Source: CAD feature listing. Evaluate the final solid. Frame: model axes, mm. A direction names the side the tool comes from. Give positions to 0.01 mm unless a question says otherwise; leave off trailing zeros. Order: outer loops, then holes, each group sorted by start corner. A loop starts at its lowest first (then second) coordinate and runs counter-clockwise, first axis right, second up. Notation, with made-up numbers: (38.25, 72.25) - (62.25, 72.25) arc R13 ccw to (62.25, 81.25) - close; hole circle Ø9 at (-36.5, -2.5). An arc over 180 degrees is marked (long way). Write each question's results on one line, items separated by ' | '. Start each with the question number.
Item 1: Set-up query: faces 4 (the cylindrical face through (-41.205, 1.768, 26.863)), 5 (the flat face through (0, -5, -48)), 6 (the cylindrical face through (1.245, -2.465, 53.502)). Return all of +Z, -Z, +X, -X, +Y, -Y with unobstructed straight access to the full face (end or side cutting, diameter ignored); none if empty.
Item 2: Section C-C on z = -50.5. Output: boundary loops of the cut face in (x, y), and give its area (3 significant figures).
Item 3: Mould query, pull axis X, two halves, no side actions, for faces 1 (the cylindrical face through (1.245, -2.465, -47.498)), 2 (the flat face through (0, -5, 53)), 3 (the cylindrical face through (-40.56, -2.46, 24.55)). Classes: released by +X, released by -X, zero draft, split by the parting line, or undercut.
Item 4: Section D-D on x = -31.5. Output: boundary loops of the cut face in (y, z).
Item 5: Contact query for flat-ended pins moving along their axis: pin 1 Ø4.5 at (x, z) = (43.73, -25.25) entering from -Y; pin 2 Ø6 at (x, z) = (-20.5, 11) entering from -Y; pin 3 Ø4 at (x, y) = (-44.5, 1) entering from -Z; pin 4 Ø1.5 at (y, z) = (0, -27) entering from +X. Output: stop coordinate, or through.
Item 6: Line query: line 1 along X through (y, z) = (-3.9, 25.25); line 2 along X through (y, z) = (-2.4, 50.5); line 3 along Z through (x, y) = (-44.5, 2). Output: solid intervals per line, ascending.
Item 7: Section B-B on z = -3. Output: boundary loops of the cut face in (x, y).
Item 8: Section A-A on y = -3.25. State how many separate pieces and enclosed holes the cut face has, and give its area (3 significant figures).
```python
from build123d import *

# Parameters (mm, degrees)
SKETCH1_R           = 57
BOSS_EXTRUDE1_DEPTH = 3
SKETCH2_R           = 2
CUT_EXTRUDE1_DEPTH  = 81.665977958
CIRPATTERN1_COUNT   = 6
SKETCH5_R           = 3.25
BOSS_EXTRUDE2_DEPTH = 5
SKETCH4_R           = 16.5
CUT_EXTRUDE3_DEPTH  = 81.765091469
SKETCH8_R           = 2
CUT_EXTRUDE4_DEPTH  = 82.006172604
SKETCH9_R           = 3
CUT_EXTRUDE5_DEPTH  = 2.5


with BuildPart() as part:
    # Sketch1 → Boss-Extrude1 (new body)
    with BuildSketch(Plane(origin=(0, 0, 0), x_dir=(1, 0, 0), z_dir=(0, 1, 0))):
        with Locations(Location((0, 0, 0), (0, 0, 270))):
            Circle(SKETCH1_R)
    extrude(amount=BOSS_EXTRUDE1_DEPTH)

    # Sketch2 → Cut-Extrude1 (cut, through all)
    with BuildSketch(Plane(origin=(0, 3, 0), x_dir=(1, 0, 0), z_dir=(0, 1, 0))):
        with Locations(Location((0, 50.5, 0), (0, 0, 270))):
            Circle(SKETCH2_R)
    cut_extrude1 = extrude(amount=-CUT_EXTRUDE1_DEPTH, mode=Mode.SUBTRACT)

    # CirPattern1: Cut-Extrude1 ×6 about axis
    cirpattern1_axis = Axis((0, 0, 0), (0, 1, 0))
    for i in range(1, CIRPATTERN1_COUNT):
        add(cut_extrude1.rotate(cirpattern1_axis, i * 360 / CIRPATTERN1_COUNT), mode=Mode.SUBTRACT)

    # Sketch5 → Boss-Extrude2 (add)
    with BuildSketch(Plane.XZ):
        with Locations(Location((0, 50.5, 0), (0, 0, 90))):
            Circle(SKETCH5_R)
        with Locations(Location((43.734282891, 25.25, 0), (0, 0, 90))):
            Circle(SKETCH5_R)
        with Locations(Location((43.734282891, -25.25, 0), (0, 0, 90))):
            Circle(SKETCH5_R)
        with Locations(Location((0, -50.5, 0), (0, 0, 90))):
            Circle(SKETCH5_R)
        with Locations(Location((-43.734282891, -25.25, 0), (0, 0, 90))):
            Circle(SKETCH5_R)
        with Locations(Location((-43.734282891, 25.25, 0), (0, 0, 90))):
            Circle(SKETCH5_R)
    extrude(amount=BOSS_EXTRUDE2_DEPTH)

    # Sketch4 → Cut-Extrude3 (cut, through all)
    with BuildSketch(Plane.XZ):
        with Locations(Location((0, 0, 0), (0, 0, 270))):
            Circle(SKETCH4_R)
    extrude(amount=-CUT_EXTRUDE3_DEPTH, mode=Mode.SUBTRACT)

    # Sketch8 → Cut-Extrude4 (cut, through all)
    with BuildSketch(Plane(origin=(0, 3, 0), x_dir=(1, 0, 0), z_dir=(0, 1, 0))):
        with Locations(Location((-43.734282891, -25.25, 0), (0, 0, 270))):
            Circle(SKETCH8_R)
        with Locations(Location((0, -50.5, 0), (0, 0, 270))):
            Circle(SKETCH8_R)
        with Locations(Location((43.734282891, -25.25, 0), (0, 0, 270))):
            Circle(SKETCH8_R)
        with Locations(Location((43.734282891, 25.25, 0), (0, 0, 270))):
            Circle(SKETCH8_R)
        with Locations(Location((0, 50.5, 0), (0, 0, 270))):
            Circle(SKETCH8_R)
        with Locations(Location((-43.734282891, 25.25, 0), (0, 0, 270))):
            Circle(SKETCH8_R)
    extrude(amount=-CUT_EXTRUDE4_DEPTH, mode=Mode.SUBTRACT)

    # Sketch9 → Cut-Extrude5 (cut)
    with BuildSketch(Plane(origin=(0, 3, 0), x_dir=(1, 0, 0), z_dir=(0, 1, 0))):
        with Locations(Location((-43.734282891, 25.25, 0), (0, 0, 270))):
            Circle(SKETCH9_R)
        with Locations(Location((0, 50.5, 0), (0, 0, 270))):
            Circle(SKETCH9_R)
        with Locations(Location((43.734282891, 25.25, 0), (0, 0, 270))):
            Circle(SKETCH9_R)
        with Locations(Location((43.734282891, -25.25, 0), (0, 0, 270))):
            Circle(SKETCH9_R)
        with Locations(Location((0, -50.5, 0), (0, 0, 270))):
            Circle(SKETCH9_R)
        with Locations(Location((-43.734282891, -25.25, 0), (0, 0, 270))):
            Circle(SKETCH9_R)
    extrude(amount=-CUT_EXTRUDE5_DEPTH, mode=Mode.SUBTRACT)


solid = part.part
```
Evaluation:
1) face 4: +Y | face 5: +Z, -Z, +X, -X, -Y | face 6: -Y
2) outline: (-26.43, 0) - (-3.25, 0) - (-3.25, -5) - (-2, -5) - (-2, 0.5) - (-3, 0.5) - (-3, 3) - (-26.43, 3) - close; (2, -5) - (3.25, -5) - (3.25, 0) - (26.43, 0) - (26.43, 3) - (3, 3) - (3, 0.5) - (2, 0.5) - close | area: 154 mm^2
3) face 1: split by the parting line | face 2: zero draft | face 3: undercut
4) outline: (0, -47.51) - (3, -47.51) - (3, 47.51) - (0, 47.51) - close
5) pin 1: stops at y = -5 | pin 2: stops at y = 0 | pin 3: stops at z = -37.98 | pin 4: stops at x = 50.6
6) line 1: x = -46.98 to -45.73, -41.73 to -40.48, 40.48 to 41.73, 45.73 to 46.98 | line 2: x = -3.25 to -2, 2 to 3.25 | line 3: z = -35.62 to -28.15, -22.35 to 22.35, 28.15 to 35.62
7) outline: (-56.92, 0) - (-16.22, 0) - (-16.22, 3) - (-56.92, 3) - close; (16.22, 0) - (56.92, 0) - (56.92, 3) - (16.22, 3) - close
8) separate pieces: 6 | enclosed holes: 6 | area: 124 mm^2
